Here's how the part is built. I have some questions about the finished solid (model axes, mm). A direction names the side the tool comes from. Round coordinates to 2 decimals unless told otherwise and drop trailing zeros. Order: outer loops, then holes, each group sorted by start corner. A loop starts at its lowest first (then second) coordinate and runs counter-clockwise, first axis right, second up. Notation, with made-up numbers: (-7, 80.5) -> (43, 80.5) arc R16 ccw to (43, 97.5) -> close; hole circle Ø6 at (-23.5, 35.5). An arc over 180 degrees is marked (long way). Use a Markdown table: item, result. Add a question column.
(1) I want a section at A-A, the plane y = 58.5. Please give me the cut outline in (x, z).
(2) On a 3-axis mill with a long thin cutter (end or side, diameter ignored), from which of +Z, -Z, +X, -X, +Y, -Y can I reach the whole of each face in a straight line? I mean faces 4 (the face through (-9.248, 74.287, 1.521)), 5 (the face through (3, -74, 1)), 6 (the face through (-2, 51, 1)). Say none if no direction works.
(3) If I drill on probe 1 along X at (y, z) = (-55, 0.95); probe 2 along Y at (x, z) = (4, 2.3); probe 3 along Y at (x, z) = (-3.75, 1.65), over which ranges is the centre line in solid material (lowest first)?
(4) Thinking about a two-plate mould opening in X: for faces 1 (the face through (9.287, 74.248, 1.521)), 2 (the face through (-9.287, -74.248, 1.521)), 3 (the face through (-2.5, -63, 2)), which applies, pulls with the +X half, pulls with the -X half, needs draft (parallel to the pull), parting line crosses it, or undercut?
Autodesk Inventor part; units mm, degrees
ref_plane "YZ Plane" through (0, 0, 0) normal (1, 0, 0) x (0, 1, 0)
ref_plane "XZ Plane" through (0, 0, 0) normal (0, 1, 0) x (-1, 0, 0)
ref_plane "XY Plane" through (0, 0, 0) normal (0, 0, 1) x (1, 0, 0)
sketch "Sketch1" plane through (0, 0, 0) normal (0, 0, 1) x (1, 0, 0)
  line L0 (-10, -75) -> (10, -75)
  line L1 (10, -75) -> (10, 75)
  line L2 (10, 75) -> (-10, 75)
  line L3 (-10, 75) -> (-10, -75)
  line L4 (-10, -75) -> (10, 75) construction
  line L5 (10, -75) -> (-10, 75) construction
  point P0 (0, 0)
  dimension "d0" = 20
  dimension "d1" = 150
extrude "Extrusion1" add sketch "Sketch1" along normal blind 3
sketch "Sketch2" plane through (0, 0, 3) normal (0, 0, 1) x (1, 0, 0)
  line L0 (0, -105) -> (0, 105) construction
  line L1 (-2.5, 50) -> (2.5, 50)
  line L2 (2.5, 50) -> (2.5, 75)
  line L3 (2.5, 75) -> (-2.5, 75)
  line L4 (-2.5, 75) -> (-2.5, 50)
  line L5 (-2.5, 50) -> (2.5, 75) construction
  line L6 (2.5, 50) -> (-2.5, 75) construction
  line L7 (10, 75) -> (-10, 75) construction
  line L8 (-14, 0) -> (14, 0)
  line L9 (-2.5, -50) -> (2.5, -50)
  line L10 (2.5, -50) -> (2.5, -75)
  line L11 (2.5, -75) -> (-2.5, -75)
  line L12 (-2.5, -75) -> (-2.5, -50)
  line L13 (-2.5, -50) -> (2.5, -75) construction
  line L14 (2.5, -50) -> (-2.5, -75) construction
  line L15 (10, -75) -> (-10, -75) construction
  point P0 (0, 0)
  point P1 (0, 62.5)
  point P2 (0, 75)
  point P3 (0, -62.5)
  point P4 (0, -75)
  dimension "d4" = 100
  dimension "d5" = 5
extrude "Extrusion2" cut sketch "Sketch2" against normal blind 3
fillet "Fillet1" radius 2.5 12 edges at (-2.5, 50, 1.5) (2.5, 50, 1.5) (-2.5, 75, 1.5) (2.5, 75, 1.5) (10, 75, 1.5) (-10, 75, 1.5) (10, -75, 1.5) (-10, -75, 1.5) (-2.5, -75, 1.5) (2.5, -75, 1.5) (-2.5, -50, 1.5) (2.5, -50, 1.5)
sketch "Sketch3" plane through (0, 0, 3) normal (0, 0, 1) x (1, 0, 0)
  arc A0 (2.5, -72.5) -> (5, -75) centre (5, -72.5) ccw
  line L0 (5, -75) -> (7.5, -75)
  arc A1 (7.5, -75) -> (10, -72.5) centre (7.5, -72.5) ccw
  line L1 (10, -72.5) -> (10, 72.5)
  arc A2 (10, 72.5) -> (7.5, 75) centre (7.5, 72.5) ccw
  line L2 (7.5, 75) -> (5, 75)
  arc A3 (5, 75) -> (2.5, 72.5) centre (5, 72.5) ccw
  line L3 (2.5, 72.5) -> (2.5, 52.5)
  arc A4 (-2.5, 52.5) -> (2.5, 52.5) centre (0, 52.5) ccw
  line L4 (-2.5, 52.5) -> (-2.5, 72.5)
  arc A5 (-2.5, 72.5) -> (-5, 75) centre (-5, 72.5) ccw
  line L5 (-5, 75) -> (-7.5, 75)
  arc A6 (-7.5, 75) -> (-10, 72.5) centre (-7.5, 72.5) ccw
  line L6 (-10, 72.5) -> (-10, -72.5)
  arc A7 (-10, -72.5) -> (-7.5, -75) centre (-7.5, -72.5) ccw
  line L7 (-7.5, -75) -> (-5, -75)
  arc A8 (-5, -75) -> (-2.5, -72.5) centre (-5, -72.5) ccw
  line L8 (-2.5, -72.5) -> (-2.5, -52.5)
  arc A9 (2.5, -52.5) -> (-2.5, -52.5) centre (0, -52.5) ccw
  line L9 (2.5, -52.5) -> (2.5, -72.5)
  point P0 (0, 0)
properties part number "LED_Glass"
Taken from the geometry:
| question | item | result |
|---|---|---|
| 1 | outline | (-10, 0) -> (-2.5, 0) -> (-2.5, 3) -> (-10, 3) -> close; (2.5, 0) -> (10, 0) -> (10, 3) -> (2.5, 3) -> close |
| 2 | face 4 | +Z, -Z, -X, +Y |
| 2 | face 5 | +Z, -Z, -Y |
| 2 | face 6 | +Z, -Z, +Y |
| 3 | probe 1 | x = -10 to -2.5, 2.5 to 10 |
| 3 | probe 2 | y = -74.79 to 74.79 |
| 3 | probe 3 | y = -74.67 to 74.67 |
| 4 | face 1 | pulls with the +X half |
| 4 | face 2 | pulls with the -X half |
| 4 | face 3 | undercut |
